Answer from the drawing. Dimensions are ordinates in mm from the lowest x, y and z of the part. A direction names the side the tool comes from. Give positions to 0.01 mm unless a question says otherwise; leave off trailing zeros. Order: outer loops, then holes, each group sorted by start corner. A loop starts at its lowest first (then second) coordinate and runs counter-clockwise, first axis right, second up.
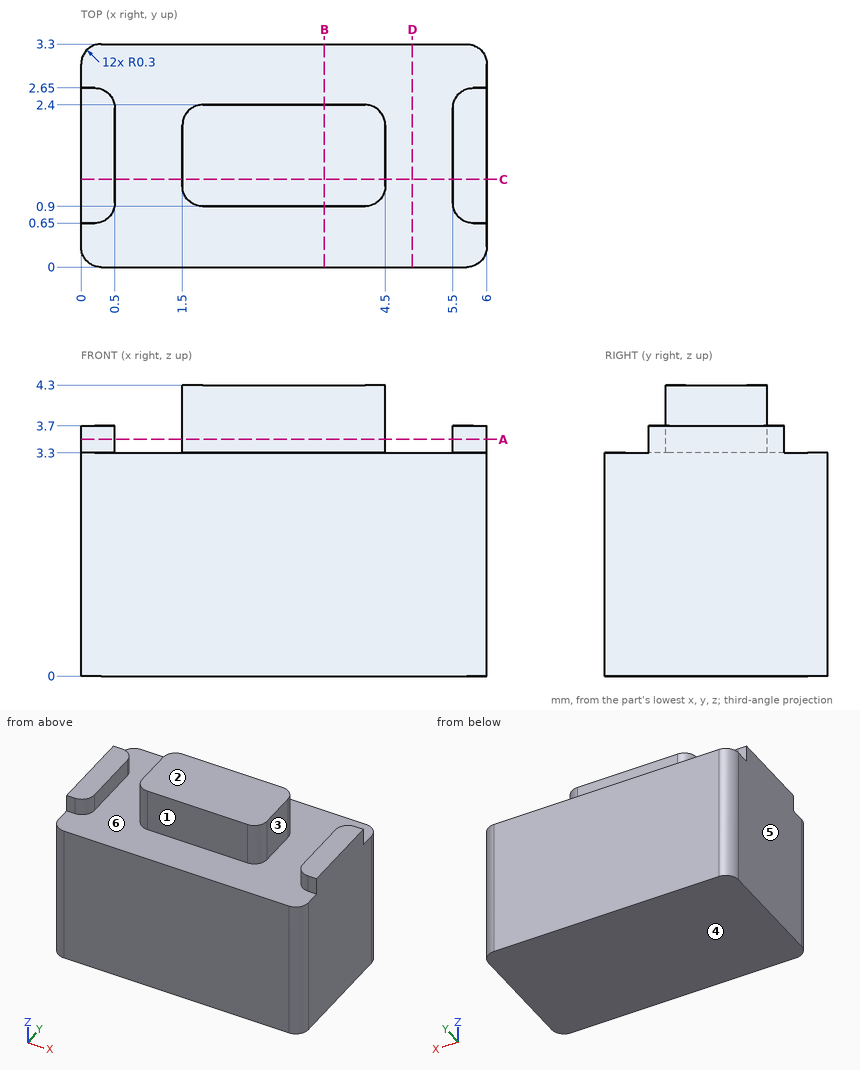
1) A tool of negligible diameter and unlimited length cuts with its end or side. For the marked faces 1 and 2, from which of +Z, -Z, +X, -X, +Y, -Y can it reach the whole face along a straight path? Write none if from no direction.
Final values:
face 1: +Z, -Y
face 2: +Z, +X, -X, +Y, -Y
2) For a pull along X with two mould halves and no side action, classify the marked faces 3, 4, 5 and 6 as released by +X, released by -X, zero draft, split by the parting line, or undercut.
Final values:
face 3: undercut
face 4: zero draft
face 5: released by -X
face 6: undercut
3) The part is cut by section D-D on x = 4.9. Determine the outline of the cut face in (y, z).
Final values:
outline: (0, 0) - (3.3, 0) - (3.3, 3.3) - (0, 3.3) - close
4) The part is cut by section C-C on y = 1.3. Determine the outline of the cut face in (x, z).
Final values:
outline: (0, 0) - (6, 0) - (6, 3.7) - (5.5, 3.7) - (5.5, 3.3) - (4.5, 3.3) - (4.5, 4.3) - (1.5, 4.3) - (1.5, 3.3) - (0.5, 3.3) - (0.5, 3.7) - (0, 3.7) - close
5) Consider L1, parallel to Z at x = 0.7, y = 2.85; L2, parallel to X at y = 2.1, z = 4.05; L3, parallel to Y at x = 3.8, z = 3.9. Determine where each line is inside the solid, lowest interval first.
Final values:
L1: z = 0 to 3.3
L2: x = 1.5 to 4.5
L3: y = 0.9 to 2.4
6) Given pin 1 (0.8 mm diameter, centred on x = 3.5, z = 4, fed in from -Y); pin 2 (0.6 mm diameter, centred on x = 0, y = 1.5, fed in from +Z); pin 3 (0.8 mm diameter, centred on x = 3.5, z = 4, fed in from +Y), each flat-ended and moving along its own axis, determine where each tip first touches the part or whether it passes through.
Final values:
pin 1: stops at y = 0.9
pin 2: stops at z = 3.7
pin 3: stops at y = 2.4
7) The part is cut by section B-B on x = 3.6. Determine the outline of the cut face in (y, z), and give its area (3 significant figures).
Final values:
outline: (0, 0) - (3.3, 0) - (3.3, 3.3) - (2.4, 3.3) - (2.4, 4.3) - (0.9, 4.3) - (0.9, 3.3) - (0, 3.3) - close
area: 12.4 mm2
8) The part is cut by section A-A on z = 3.5. Determine the outline of the cut face in (x, y), and give its area (3 significant figures).
Final values:
outline: (0, 0.65) - (0.2, 0.65) arc R0.3 ccw to (0.5, 0.95) - (0.5, 2.35) arc R0.3 ccw to (0.2, 2.65) - (0, 2.65) - close; (1.5, 1.2) arc R0.3 ccw to (1.8, 0.9) - (4.2, 0.9) arc R0.3 ccw to (4.5, 1.2) - (4.5, 2.1) arc R0.3 ccw to (4.2, 2.4) - (1.8, 2.4) arc R0.3 ccw to (1.5, 2.1) - close; (5.5, 0.95) arc R0.3 ccw to (5.8, 0.65) - (6, 0.65) - (6, 2.65) - (5.8, 2.65) arc R0.3 ccw to (5.5, 2.35) - close
area: 6.35 mm2
